Check sheet for the modelled part. Datum: model origin and axes. Units: mm. A direction names the side the tool comes from. Give positions to 0.01 mm unless a question says otherwise; leave off trailing zeros. Loops run counter-clockwise (first coordinate to the right, second up) from the corner with the lowest first, then second, coordinate; pieces in that order, holes last. Notation, with made-up numbers: (80.25, 88) - (132.25, 88) arc R24 cw to (132.25, 110) - close; hole circle Ø7 at (-33, 63). An arc over 180 degrees is marked (long way). Answer in a Markdown table with one row per item. Add a question column.
(1) Thickness scan on L1, parallel to Z at x = -4.5, y = 3.5; L2, parallel to Z at x = 0.75, y = -1; L3, parallel to Y at x = -0.5, z = 67.5. Record the ranges inside material, lowest first.
(2) Sectioned sample at A-A on x = -6.75. Enter the section's corners in (y, z).
(3) Draft check along Y on faces 4 (the face through (-10.68, -3.36, 25.1)), 5 (the face through (0, -3, -14.929)), 6 (the face through (0, 0, 65.371)). Enter one of: released by +Y, released by -Y, zero draft, split by the parting line, or undercut.
(4) Go/stop test with flat-tipped pins: P1, Ø10, axis at x = 6.5, z = 53.5, coming from the +Y side; P2, Ø8, axis at x = 4, z = 49.5, coming from the +Y side; P3, Ø3, axis at x = -1.5, z = 68.5, coming from the -Y side; P4, Ø1.5, axis at x = -8, z = 62.5, coming from the +Y side. Record where each tip stops, or that it passes through.
(5) Sectioned sample at D-D on y = -7.25. Enter the section's corners in (x, z), then the cut area to 3 significant figures.
(6) Sectioned sample at B-B on y = 0. Enter the section's corners in (x, z), then the cut area to 3 significant figures.
(7) Set-up check for faces 1 (the face through (-2.02, -3.16, -17.39)), 2 (the face through (-4.619, 1.915, 69.695)), 3 (the face through (2.5, -0.1, -3.1)): record each of +Z, -Z, +X, -X, +Y, -Y from which the full face is reachable in a straight line by a thin tool's end or side.
(8) Sectioned sample at C-C on x = 0. State how many separate pieces and enclosed holes the cut face has, then the cut area to 3 significant figures.
from build123d import *

# Parameters (mm, degrees)
CHAMFER_1_SIZE      = 0.5
SKETCH_3_W          = 16
SKETCH_3_H          = 3
CUT_EXTRUDE_1_DEPTH = 10
SKETCH_4_R          = 1.5
CUT_EXTRUDE_2_DEPTH = 11
FILLET_1_R          = 1
SKETCH_5_R          = 9
EXTRUDE_1_DEPTH     = 1


with BuildPart() as part:
    # 草图1 → 旋转1 (revolve)
    with BuildSketch(Plane(origin=(0, 0, 0), x_dir=(1, 0, 0), z_dir=(0, 1, 0)), mode=Mode.PRIVATE) as revolve_1_sk:
        Polygon((2.5, 14.928900778), (2.5, -8.371099222), (11.195443228, -8.371099222), (11.195443228, -41.371099222), (5, -41.371099222), (5, -75.371099222), (0, -75.371099222), (0, 20.928900778), (2.5, 20.928900778), (3.75, 20.928900778), (3.75, 14.928900778), align=None)
    revolve(revolve_1_sk.sketch.rotate(Axis((0, 0, -46.113181398), (0, 0, 1)), 180), axis=Axis((0, 0, -46.113181398), (0, 0, 1)))

    # 倒角1
    chamfer_1_edges = [part.edges().sort_by_distance(p)[0] for p in [
        (5, 0, 75.371099222),
    ]]
    chamfer(chamfer_1_edges, length=CHAMFER_1_SIZE)

    # 草图3 → 切除-拉伸1 (cut)
    with BuildSketch(Plane.XY.offset(75.371099222)):
        Rectangle(SKETCH_3_W, SKETCH_3_H)
    extrude(amount=-CUT_EXTRUDE_1_DEPTH, mode=Mode.SUBTRACT)

    # 草图4 → 切除-拉伸2 (cut, symmetric)
    with BuildSketch(Plane(origin=(0, 0, 0), x_dir=(1, 0, 0), z_dir=(0, 1, 0))):
        with Locations(Location((0, -71.371099222, 0), (0, 0, 90))):
            Circle(SKETCH_4_R)
    extrude(amount=CUT_EXTRUDE_2_DEPTH, both=True, mode=Mode.SUBTRACT)

    # 圆角1
    fillet_1_edges = [part.edges().sort_by_distance(p)[0] for p in [
        (3.75, 0, -20.928900778),
    ]]
    fillet(fillet_1_edges, radius=FILLET_1_R)

    # 草图5 → 凸台-拉伸1 (add)
    with BuildSketch(Plane.XY.offset(64.371099222)):
        Circle(SKETCH_5_R)
    extrude(amount=-EXTRUDE_1_DEPTH)


solid = part.part
Reply:
| question | item | result |
|---|---|---|
| 1 | L1 | 8.37 to 41.37, 63.37 to 64.37 |
| 1 | L2 | -20.93 to 65.37 |
| 1 | L3 | -4.97 to -1.5, 1.5 to 4.97 |
| 2 | outline | (-8.93, 8.37) - (8.93, 8.37) - (8.93, 41.37) - (-8.93, 41.37) - close; (-5.95, 63.37) - (5.95, 63.37) - (5.95, 64.37) - (-5.95, 64.37) - close |
| 3 | face 4 | split by the parting line |
| 3 | face 5 | zero draft |
| 3 | face 6 | undercut |
| 4 | P1 | y = 4.77 |
| 4 | P2 | y = 5 |
| 4 | P3 | y = -5 |
| 4 | P4 | through |
| 5 | outline | (-8.53, 8.37) - (8.53, 8.37) - (8.53, 41.37) - (-8.53, 41.37) - close; (-5.33, 63.37) - (5.33, 63.37) - (5.33, 64.37) - (-5.33, 64.37) - close |
| 5 | area | 574 mm^2 |
| 6 | outline | (-11.2, 8.37) - (-2.5, 8.37) - (-2.5, -14.93) - (-3.75, -14.93) - (-3.75, -19.93) arc R1 ccw to (-2.75, -20.93) - (2.75, -20.93) arc R1 ccw to (3.75, -19.93) - (3.75, -14.93) - (2.5, -14.93) - (2.5, 8.37) - (11.2, 8.37) - (11.2, 41.37) - (5, 41.37) - (5, 63.37) - (9, 63.37) - (9, 64.37) - (5, 64.37) - (5, 65.37) - (-5, 65.37) - (-5, 64.37) - (-9, 64.37) - (-9, 63.37) - (-5, 63.37) - (-5, 41.37) - (-11.2, 41.37) - close |
| 6 | area | 1,150 mm^2 |
| 7 | face 1 | -Z |
| 7 | face 2 | +Z |
| 7 | face 3 | none |
| 8 | separate pieces | 3 |
| 8 | enclosed holes | 0 |
| 8 | area | 1,200 mm^2 |
